Design review of the part built by this model. Coordinates are the model's own, in mm. Face numbers are marked on the shaded views. Coordinates: 2 decimals unless noted, no trailing zeros. Order: outer loops, then holes, each group sorted by start corner. A loop starts at its lowest first (then second) coordinate and runs counter-clockwise, first axis right, second up. Notation, with made-up numbers: M -18.5,-21.5 L 38.5,-21.5 A18 ccw 38.5,0.5 Z; hole C 49,-13 d8. An arc over 180 degrees is marked long. Use CSV: the item, a comma, the result in double quotes.
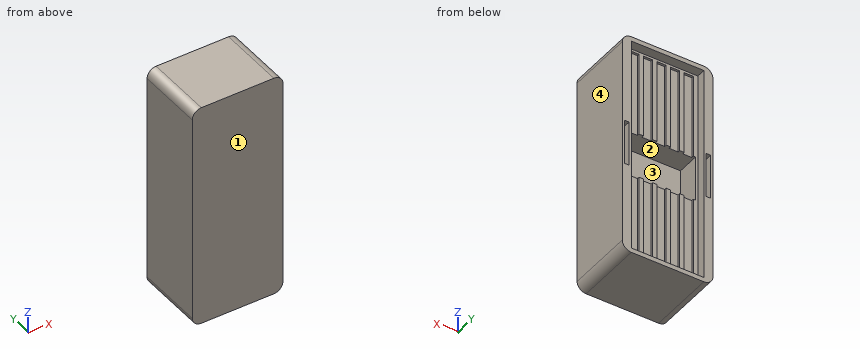
Autodesk Inventor part; units mm, degrees
ref_plane "YZ Plane" through (0, 0, 0) normal (1, 0, 0) x (0, 1, 0)
ref_plane "XZ Plane" through (0, 0, 0) normal (0, 1, 0) x (-1, 0, 0)
ref_plane "XY Plane" through (0, 0, 0) normal (0, 0, 1) x (1, 0, 0)
sketch "Skizze1" plane through (0, 0, 0) normal (0, 1, 0) x (-1, 0, 0)
  line L0 (10, 25) -> (-10, 25)
  line L1 (-10, 25) -> (-10, -25)
  line L2 (-10, -25) -> (10, -25)
  line L3 (10, -25) -> (10, 25)
  point P0 (0, 0)
  dimension "d0" = 50
  dimension "d1" = 20
  dimension "d20" = 10
  dimension "d21" = 25
extrude "Extrusion1" add sketch "Skizze1" along normal blind 15
sketch "Skizze3" plane through (0, 15, 0) normal (0, 1, 0) x (1, 0, 0)
  line L0 (-8, 24) -> (8, 24)
  line L1 (8, 24) -> (8, -24)
  line L2 (8, -24) -> (-8, -24)
  line L3 (-8, -24) -> (-8, 24)
  line L4 (10, 25) -> (-10, 25)
  line L5 (-10, -25) -> (10, -25)
  line L6 (10, -25) -> (10, 25)
  line L7 (-10, 25) -> (-10, -25)
  point P0 (0, 0)
  dimension "d4" = 1
  dimension "d5" = 1
  dimension "d6" = 2
  dimension "d7" = 2
extrude "Extrusion2" cut sketch "Skizze3" against normal blind 2 contours L0 L1 L2 L3
sketch "Skizze4" plane through (0, 13, 0) normal (0, 1, 0) x (1, 0, 0)
  line L0 (-1, 23.5) -> (1, 23.5)
  line L1 (1, 23.5) -> (1, -23.5)
  line L2 (1, -23.5) -> (-1, -23.5)
  line L3 (-1, -23.5) -> (-1, 23.5)
  line L4 (-8, 24) -> (8, 24)
  line L5 (8, -24) -> (-8, -24)
  line L6 (2, 23.5) -> (4, 23.5)
  line L7 (4, 23.5) -> (4, -23.5)
  line L8 (4, -23.5) -> (2, -23.5)
  line L9 (2, -23.5) -> (2, 23.5)
  line L10 (-7, 23.5) -> (-5, 23.5)
  line L11 (-5, 23.5) -> (-5, -23.5)
  line L12 (-5, -23.5) -> (-7, -23.5)
  line L13 (-7, -23.5) -> (-7, 23.5)
  line L14 (-4, 23.5) -> (-2, 23.5)
  line L15 (-2, 23.5) -> (-2, -23.5)
  line L16 (-2, -23.5) -> (-4, -23.5)
  line L17 (-4, -23.5) -> (-4, 23.5)
  line L18 (5, 23.5) -> (7, 23.5)
  line L19 (7, 23.5) -> (7, -23.5)
  line L20 (7, -23.5) -> (5, -23.5)
  line L21 (5, -23.5) -> (5, 23.5)
  line L22 (-8, -24) -> (-8, 24)
  line L23 (8, 24) -> (8, -24)
  point P0 (0, 0)
  point P1 (0, -23.5)
  point P2 (0, -24)
  point P3 (6, 23.5)
  dimension "d10" = 2
  dimension "d11" = 0.5
  dimension "d12" = 0.5
  dimension "d33" = 2
  dimension "d34" = 2
  dimension "d35" = 2
  dimension "d36" = 2
  dimension "d37" = 1
  dimension "d38" = 1
  dimension "d39" = 1
  dimension "d40" = 1
  dimension "d41" = 1
  dimension "d42" = 1
  dimension "d50" = 47
  dimension "d51" = 0.5
  dimension "d52" = 0.5
  dimension "d53" = 0.5
  dimension "d54" = 0.5
  dimension "d55" = 47
sketch "Skizze5" plane through (0, 0, 0) normal (1, 0, 0) x (0, 1, 0)
  point P0 (0, 0)
extrude "Extrusion3" cut sketch "Skizze4" against normal blind 0.5 contours L0 L1 L2 L3 | L6 L7 L8 L9 | L10 L11 L12 L13 | L14 L15 L16 L17 | L18 L19 L20 L21
sketch "Skizze6" plane through (0, 13, 0) normal (0, 1, 0) x (1, 0, 0)
  line L0 (8, 24) -> (8, -24)
  point P0 (0, 0)
  point P1 (4.1748, -18.2105)
  point P2 (-0.1937, 19)
  point P3 (8, 0)
sketch "Skizze8" plane through (0, 15, 0) normal (0, 1, 0) x (1, 0, 0)
  point P0 (0, 0)
sketch "Skizze9" plane through (0, 15, 0) normal (0, 1, 0) x (1, 0, 0)
  line L0 (9.5, 5) -> (8.5, 5)
  line L1 (8.5, 5) -> (8.5, -5)
  line L2 (8.5, -5) -> (9.5, -5)
  line L3 (9.5, -5) -> (9.5, 5)
  line L4 (8, 24) -> (8, -24) construction
  line L5 (-8.5, -5) -> (-9.5, -5)
  line L6 (-9.5, -5) -> (-9.5, 5)
  line L7 (-9.5, 5) -> (-8.5, 5)
  line L8 (-8.5, 5) -> (-8.5, -5)
  line L9 (-10, 25) -> (-10, -25)
  point P0 (0, 0)
  point P1 (9, -5)
  point P2 (9.5, 0)
  dimension "d23" = 10
  dimension "d24" = 0.5
  dimension "d25" = 1
  dimension "d26" = 0
  dimension "d29" = 1
  dimension "d30" = 0.5
extrude "Extrusion5" cut sketch "Skizze9" against normal blind 5
sketch "Skizze10" plane through (0, 13, 0) normal (0, 1, 0) x (1, 0, 0)
  line L0 (-7.5, 5) -> (7.5, 5)
  line L1 (7.5, 5) -> (7.5, -5)
  line L2 (7.5, -5) -> (-7.5, -5)
  line L3 (-7.5, -5) -> (-7.5, 5)
  line L4 (-8, -24) -> (-8, 24)
  line L5 (8, 24) -> (8, -24)
  line L6 (-8, 24) -> (8, 24)
  point P0 (0, 0)
  dimension "d43" = 0.5
  dimension "d44" = 0.5
  dimension "d45" = 10
  dimension "d46" = 19
extrude "Extrusion6" cut sketch "Skizze10" against normal blind 5
fillet "Rundung1" radius 2 4 edges at (10, 7.5, 25) (-10, 7.5, 25) (10, 7.5, -25) (-10, 7.5, -25)
properties part number "Nadelbox"
(1) Add section C-C on x = -3. State the section outline as (y, z) points.
The answers:
outline,"M 0,-25 L 15,-25 L 15,-24 L 13,-24 L 13,-23.5 L 12.5,-23.5 L 12.5,-5 L 8,-5 L 8,5 L 12.5,5 L 12.5,23.5 L 13,23.5 L 13,24 L 15,24 L 15,25 L 0,25 Z"
(2) Wall thickness on probe 1 along X at (y, z) = (12.25, -3.5); probe 2 along X at (y, z) = (12.75, -13.5); probe 3 along X at (y, z) = (8.5, 0.5): over which ranges is each line inside the solid? List them lowest first.
The answers:
probe 1,"x = -10 to -9.5, -8.5 to -7.5, 7.5 to 8.5, 9.5 to 10"
probe 2,"x = -10 to -7, -5 to -4, -2 to -1, 1 to 2, 4 to 5, 7 to 10"
probe 3,"x = -10 to -7.5, 7.5 to 10"
(3) Add section A-A on y = 10.5. State the section outline as (x, z) points.
The answers:
outline,"M -10,-23 A2 ccw -8,-25 L 8,-25 A2 ccw 10,-23 L 10,23 A2 ccw 8,25 L -8,25 A2 ccw -10,23 Z; hole M -9.5,-5 L -8.5,-5 L -8.5,5 L -9.5,5 Z; hole M -7.5,-5 L 7.5,-5 L 7.5,5 L -7.5,5 Z; hole M 8.5,-5 L 9.5,-5 L 9.5,5 L 8.5,5 Z"
(4) The part is to be moulded in two halves that separate along X. For the marked faces 1, 2, 3 and 4, say which applies: pulls with the +X half, pulls with the -X half, needs draft (parallel to the pull), parting line crosses it, or undercut.
The answers:
face 1,"needs draft"
face 2,"undercut"
face 3,"undercut"
face 4,"pulls with the +X half"
(5) Add section D-D on y = 13.5. State the section outline as (x, z) points, and give its area (3 significant figures).
The answers:
outline,"M -10,-23 A2 ccw -8,-25 L 8,-25 A2 ccw 10,-23 L 10,23 A2 ccw 8,25 L -8,25 A2 ccw -10,23 Z; hole M -9.5,-5 L -8.5,-5 L -8.5,5 L -9.5,5 Z; hole M -8,-24 L 8,-24 L 8,24 L -8,24 Z; hole M 8.5,-5 L 9.5,-5 L 9.5,5 L 8.5,5 Z"
area,"209 mm2"
(6) Clearance check with flat-ended pins moving along their axes: P1, Ø1.1, axis at x = -9, y = 12, coming from the +Z side; P2, Ø1, axis at x = -6, z = -17.5, coming from the +Y side. State where each tip first meets the part, or that it passes through.
The answers:
P1,"stops at z = 24.95"
P2,"stops at y = 12.5"
(7) Add section B-B on z = -10. State the section outline as (x, y) points.
The answers:
outline,"M -10,0 L 10,0 L 10,15 L 8,15 L 8,13 L 7,13 L 7,12.5 L 5,12.5 L 5,13 L 4,13 L 4,12.5 L 2,12.5 L 2,13 L 1,13 L 1,12.5 L -1,12.5 L -1,13 L -2,13 L -2,12.5 L -4,12.5 L -4,13 L -5,13 L -5,12.5 L -7,12.5 L -7,13 L -8,13 L -8,15 L -10,15 Z"
